Source: CAD feature listing. Evaluate the final solid. Frame: model axes, mm. Give positions to 0.01 mm unless a question says otherwise; leave off trailing zeros. Order: outer loops, then holes, each group sorted by start corner. A loop starts at its lowest first (then second) coordinate and runs counter-clockwise, first axis right, second up. Notation, with made-up numbers: M -36,33.25 L -22,33.25 A18 ccw -22,59.25 Z; hole C -16,34.25 d10. An arc over 180 degrees is marked long. Use CSV: the item, a comma, the result in double quotes. Start each with the question number.
1. Mould query, pull axis Z, two halves, no side actions, for faces 1 (the cylindrical face through (-1.617, 1.947, 0.67)), 2 (the cylindrical face through (22.745, 1.996, 5.361)), 3 (the cylindrical face through (23, 2, 0)), 4 (the flat face through (0, 2, -7.5)). Classes: released by +Z, released by -Z, zero draft, split by the parting line, or undercut.
2. Line query: line 1 along X through (y, z) = (2.3, 1); line 2 along Z through (x, y) = (-21.5, 1.65); line 3 along X through (y, z) = (1.1, -6). Output: solid intervals per line, ascending. Write a range as [from, to].
3. Section query A-A, the plane x = 0. Return the cut outline in (y, z).
4. Section query B-B, the plane y = 2.05. State how many separate pieces and enclosed holes the cut face has, plus the area to 3 significant figures.
Autodesk Inventor part; units mm, degrees
ref_plane "YZ Plane" through (0, 0, 0) normal (1, 0, 0) x (0, 1, 0)
ref_plane "XZ Plane" through (0, 0, 0) normal (0, 1, 0) x (-1, 0, 0)
ref_plane "XY Plane" through (0, 0, 0) normal (0, 0, 1) x (1, 0, 0)
sketch "Sketch1" plane through (0, 0, 0) normal (0, 1, 0) x (-1, 0, 0)
  line L0 (25, -7.5) -> (-25, -7.5)
  line L1 (-25, -7.5) -> (-25, 7.5)
  line L2 (-25, 7.5) -> (25, 7.5)
  line L3 (25, 7.5) -> (25, -7.5)
  circle A0 centre (0, 0) radius 1.75
  circle A1 centre (-21.5, 0) radius 1.5
  line L4 (0, 11.4467) -> (0, -17.1004)
  circle A2 centre (21.5, 0) radius 1.5
  point P0 (0, -7.5)
  dimension "d0" = 15
  dimension "d1" = 50
  dimension "d2" = 25
  dimension "d3" = 3.5
  dimension "d4" = 7.5
  dimension "d7" = 3
  dimension "d9" = 7.5
  dimension "d10" = 2
extrude "Extrusion2" add sketch "Sketch1" along normal blind 3.95 contours L0 L4 A0 L2 L3 | L0 L1 L2 L4 A0
fillet "Fillet1" radius 7.5 4 edges at (25, 1.975, 7.5) (25, 1.975, -7.5) (-25, 1.975, 7.5) (-25, 1.975, -7.5)
fillet "Fillet2" radius 0.5 8 edges at (22.8033, 3.95, 5.3033) (0, 3.95, -7.5) (-22.8033, 3.95, 5.3033) (0, 3.95, 7.5) (22.8033, 0, 5.3033) (0, 0, -7.5) (-22.8033, 0, 5.3033) (0, 0, 7.5)
properties part number "PropConnector"
Result set:
1,face 1,"undercut"
1,face 2,"released by +Z"
1,face 3,"undercut"
1,face 4,"released by -Z"
2,line 1,"[-24.93, -22.62], [-20.38, -1.44], [1.44, 20.38], [22.62, 24.93]"
2,line 2,"[-6.34, -1.5], [1.5, 6.34]"
2,line 3,"[-22, 22]"
3,outline,"M 0,-7 A0.5 ccw 0.5,-7.5 L 3.45,-7.5 A0.5 ccw 3.95,-7 L 3.95,-1.75 L 0,-1.75 Z; M 0,1.75 L 3.95,1.75 L 3.95,7 A0.5 ccw 3.45,7.5 L 0.5,7.5 A0.5 ccw 0,7 Z"
4,separate pieces,"1"
4,enclosed holes,"3"
4,area,"678 mm2"
